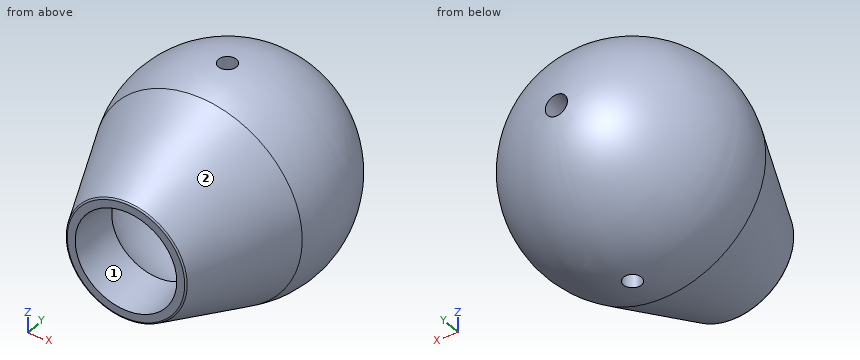
Autodesk Inventor part; units mm, degrees
ref_plane "YZ Plane" through (0, 0, 0) normal (1, 0, 0) x (0, 1, 0)
ref_plane "XZ Plane" through (0, 0, 0) normal (0, 1, 0) x (-1, 0, 0)
ref_plane "XY Plane" through (0, 0, 0) normal (0, 0, 1) x (1, 0, 0)
sketch "Skizze1" plane through (0, 0, 0) normal (0, 0, 1) x (1, 0, 0)
  line L0 (0, 104.266) -> (0, -111.9697) construction
  line L1 (-21.501, 0) -> (94.0062, 0) construction
  line L2 (6, 60.7042) -> (6, 37.6387)
  line L3 (25.2446, -55.1591) -> (27.5, -80.9387)
  line L4 (31.8318, -80.9387) -> (27.5, -80.9387)
  arc A0 (56.3567, -23.3437) -> (6, 60.7042) centre (0, 0) ccw
  line L5 (56.3567, -23.3437) -> (32.7557, -80.3214)
  arc A1 (31.8318, -80.9387) -> (32.7557, -80.3214) centre (31.8318, -79.9387) ccw
  circle A2 centre (0, 0) radius 5
  arc A3 (25.2446, -55.1591) -> (6, 37.6387) centre (0, -12) ccw
  line L6 (52.114, -33.5863) -> (46.194, -31.1342) construction
  point P0 (32.5, -80.9387)
  dimension "d3" = 6
  dimension "d12" = 5
  dimension "d15" = 5
  dimension "d16" = 27.5
  dimension "d17" = 1
  dimension "d18" = 10
  dimension "d68" = 100
  dimension "d69" = 12
  dimension "d71" = 25.7796
  dimension "d72" = 23.0655
  dimension "d73" = 22.5
  dimension "d76" = 61
  dimension "d77" = 6.4078
revolve "Umdrehung1" add sketch "Skizze1" angle 360 about axis through (0, 0, 0) along (0, -1, 0) contours A0 L5 A1 L4 L3 A3 L2
extrude "Extrusion1" cut sketch "Skizze1" along normal through all both and the other way through all contours A2
sketch "Skizze3" plane through (0, 0, 0) normal (0, 0, 1) x (1, 0, 0)
  point P0 (0, 0)
properties part number "FilmLamp" material "Beton"
Verification items for the finished model (mm, model axes). Face numbers are marked on the shaded views. Coordinates: 2 decimals unless noted, no trailing zeros. Use a Markdown table: item, result.
Q1. Go/stop test with flat-tipped pins: P1, Ø2, axis at x = 11, y = -20, coming from the -Z side; P2, Ø5, axis at y = -23, z = 18, coming from the +X side; P3, Ø2, axis at x = 10.5, y = -8.5, coming from the +Z side; P4, Ø11, axis at x = 0, z = 0, coming from the -Y side. Record where each tip stops, or that it passes through.
Reply:
| item | result |
|---|---|
| P1 | stops at z = -56.96 |
| P2 | stops at x = 54.84 |
| P3 | stops at z = 59.7 |
| P4 | passes through |
Q2. Sectioned sample at A-A, the plane x = 0. Count the separate pieces of the cut face and the enclosed holes in it, plus the area to 3 significant figures.
Reply:
| item | result |
|---|---|
| separate pieces | 4 |
| enclosed holes | 0 |
| area | 4,230 mm² |
Q3. Thickness scan on line 1 (X direction, y = -71, z = 12); line 2 (X direction, y = -24, z = 39.5); line 3 (Y direction, x = 16.5, z = 30). Record the ranges inside material, lowest first.
Reply:
| item | result |
|---|---|
| line 1 | x = -34.59 to -23.77, 23.77 to 34.59 |
| line 2 | x = -39.82 to -28.21, 28.21 to 39.82 |
| line 3 | y = -76.74 to -48.44, 24.44 to 50.49 |
Q4. Draft check along Z on the marked faces 1 and 2. Enter one of: +Z half, -Z half, draft (parallel to the pull), parting line (faces both ways), or undercut.
Reply:
| item | result |
|---|---|
| face 1 | undercut |
| face 2 | parting line |
